from build123d import *

# Parameters (mm, degrees)
CYLINDER001_R     = 0.22
CYLINDER001_DEPTH = 12.7
CYLINDER_R        = 1.25
CYLINDER_DEPTH    = 11.771704


with BuildPart() as cone001:
    # Cone001 → Cone001 (revolve)
    with BuildSketch(Plane(origin=(0, 0, 11.229008), x_dir=(1, 0, 0), z_dir=(0, -1, 0))):
        Polygon((0, 0), (0.22, 0), (1.25, 1.470992), (0, 1.470992), align=None)
    revolve(axis=Axis((0, 0, 11.229008), (0, 0, 1)))


with BuildPart() as fusion001:
    # Cylinder001 → Cylinder001 (new body)
    with BuildSketch(Plane.XY):
        Circle(CYLINDER001_R)
    extrude(amount=CYLINDER001_DEPTH)

    # Fusion001: union Cone001
    add(cone001.part)


with BuildPart() as cone:
    # Cone → Cone (revolve)
    with BuildSketch(Plane.XZ):
        Polygon((0, 0), (0.6, 0), (1.25, 0.928296), (0, 0.928296), align=None)
    revolve(axis=Axis((0, 0, 0), (0, 0, 1)))


with BuildPart() as obj1:
    # Cylinder → Cylinder (new body)
    with BuildSketch(Plane.XY.offset(0.928296)):
        Circle(CYLINDER_R)
    extrude(amount=CYLINDER_DEPTH)

    # Fusion: union Cone
    add(cone.part)

    # Cut: cut Fusion001
    add(fusion001.part, mode=Mode.SUBTRACT)


solid = obj1.part
Here's how the part is built. I have some questions about the finished solid (model axes, mm). Coordinates: 2 decimals unless noted, no trailing zeros. Order: outer loops, then holes, each group sorted by start corner. A loop starts at its lowest first (then second) coordinate and runs counter-clockwise, first axis right, second up. Notation, with made-up numbers: M -2.5,74.5 L 27.5,74.5 A9 cw 27.5,85.5 Z; hole C -28.75,-2.75 d9. An arc over 180 degrees is marked long. Answer as CSV lines item,"result".
Item 1: If I drill on line 1 (Y direction, x = 0, z = 5.75); line 2 (X direction, y = -0.1, z = 12); line 3 (Y direction, x = -0.9, z = 10.75), over which ranges is the centre line in solid material (lowest first)?
Results found:
line 1,"-1.25 to -0.22, 0.22 to 1.25"
line 2,"-1.25 to -0.75, 0.75 to 1.25"
line 3,"-0.87 to 0.87"
Item 2: We'd pull the mould along Y, two halves only. Please class faces 1 (the face through (-0.27, -1.22, 6.73)), 2 (the face through (0.49, 0.15, 11.65)): +Y half, -Y half, draft (parallel to the pull), parting line (faces both ways), or undercut.
Results found:
face 1,"parting line"
face 2,"undercut"
Item 3: Imagine slicing it at A-A on y = 0. Write out the boundary of the cut face in (x, z), plus the area to 3 significant figures.
Results found:
outline,"M -1.25,0.93 L -0.6,0 L -0.22,0 L -0.22,11.23 L -1.25,12.7 Z; M 0.22,0 L 0.6,0 L 1.25,0.93 L 1.25,12.7 L 0.22,11.23 Z"
area,"24.0 mm2"
Item 4: Imagine slicing it at D-D on z = 11.75. Write out the boundary of the cut face in (x, y), plus the area to 3 significant figures.
Results found:
outline,"C 0,0 d2.5; hole C 0,0 d1.17"
area,"3.83 mm2"
Item 5: Imagine slicing it at C-C on z = 6.75. Write out the boundary of the cut face in (x, y).
Results found:
outline,"C 0,0 d2.5; hole C 0,0 d0.44"
